Source: CAD feature listing. Evaluate the final solid. Frame: model axes, mm. Face numbers are marked on the shaded views. A direction names the side the tool comes from. Coordinates: 2 decimals unless noted, no trailing zeros. Order: outer loops, then holes, each group sorted by start corner. A loop starts at its lowest first (then second) coordinate and runs counter-clockwise, first axis right, second up.
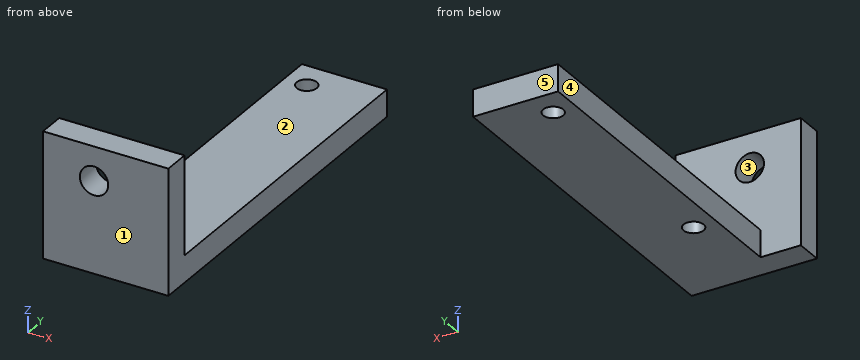
```python
from build123d import *

# Parameters (mm, degrees)
SKETCH1_W               = 10
SKETCH1_H               = 10
SKETCH1_H_2             = 65
SKETCH1_R               = 2.25
BOSS_EXTRUDE1_DEPTH     = 6
SKETCH2_W               = 28
SKETCH2_H               = 28
SKETCH2_R               = 3.175
BOSS_EXTRUDE2_DEPTH     = 6
SKETCH3_W               = 6
SKETCH3_H               = 75
BOSS_EXTRUDE3_DEPTH     = 9
SKETCH4_W               = 54.205081497
SKETCH4_H               = 103.631562047
CUT_EXTRUDE1_DEPTH      = 23
CUT_EXTRUDE1_DEPTH_BACK = 7


with BuildPart() as part:
    # Sketch1 → Boss-Extrude1 (new body)
    with BuildSketch(Plane.XY):
        with Locations((0, -37.5)):
            Rectangle(SKETCH1_W, SKETCH1_H)
        Rectangle(SKETCH1_W, SKETCH1_H_2)
        with Locations((0, 26)):
            Circle(SKETCH1_R, mode=Mode.SUBTRACT)
        with Locations((0, -26)):
            Circle(SKETCH1_R, mode=Mode.SUBTRACT)
    extrude(amount=BOSS_EXTRUDE1_DEPTH)



with BuildPart() as body_2:
    # Sketch2 → Boss-Extrude2 (new body)
    with BuildSketch(Plane.XZ.offset(42.5)):
        with Locations((0, 14)):
            Rectangle(SKETCH2_W, SKETCH2_H)
        with Locations((2.6, 20.429948245)):
            Circle(SKETCH2_R, mode=Mode.SUBTRACT)
    extrude(amount=BOSS_EXTRUDE2_DEPTH)


with BuildPart() as part_1:
    add(part.part)

    add(body_2.part)  # Boss-Extrude3 merges body 2
    # Sketch3 → Boss-Extrude3 (add)
    with BuildSketch(Plane.ZY.offset(5)):
        with Locations((3, -5)):
            Rectangle(SKETCH3_W, SKETCH3_H)
    extrude(amount=BOSS_EXTRUDE3_DEPTH)

    # Mirror1: part across plane


with BuildPart() as part_2:
    add(part_1.part)
    add(part_1.part.mirror(Plane(origin=(-14, -48.5, 0), x_dir=(0, 0, 1), z_dir=(-1, 0, 0))))

    # Sketch4 → Cut-Extrude1 (cut, two sides)
    with BuildSketch(Plane.XY.offset(6)) as cut_extrude1_sk:
        with Locations((13.102540749, -19.315781024)):
            Rectangle(SKETCH4_W, SKETCH4_H)
    extrude(amount=CUT_EXTRUDE1_DEPTH, mode=Mode.SUBTRACT)
    extrude(cut_extrude1_sk.sketch, amount=-CUT_EXTRUDE1_DEPTH_BACK, mode=Mode.SUBTRACT)


solid = part_2.part
```
1. Section query A-A, the plane y = -26. Output: boundary loops of the cut face in (x, z).
2. Contact query for flat-ended pins moving along their axis: P1, Ø2, axis at x = -17.5, y = 22.5, coming from the -Z side; P2, Ø9.5, axis at x = -23, y = -1, coming from the +Z side; P3, Ø12, axis at y = -31.5, z = 5.5, coming from the -X side. Output: stop coordinate, or through.
3. Section query B-B, the plane z = 22.25. Output: boundary loops of the cut face in (x, y).
4. Section query D-D, the plane x = -24.5. Output: boundary loops of the cut face in (y, z).
5. Draft query along X for the marked faces 3, 4 and 5. Return one class per face: +X half, -X half, draft (parallel to the pull), parting line (faces both ways), or undercut.
6. Section query C-C, the plane x = -28.5. Output: boundary loops of the cut face in (y, z).
7. Material intervals for line 1 along Y through (x, z) = (-28, 1.3); line 2 along Z through (x, y) = (-30.6, -46.6); line 3 along Y through (x, z) = (-26.25, 5.5), sorted ascending.
8. Access query for the marked faces 1 and 2. Directions: +Z, -Z, +X, -X, +Y, -Y. A direction counts if a zero-diameter tool reaches every point of the face in a straight line with its end or side. Return the directions, or none.
Answer key:
1. outline: (-33, 0) - (-30.25, 0) - (-30.25, 6) - (-33, 6) - close; (-25.75, 0) - (-14, 0) - (-14, 6) - (-25.75, 6) - close
2. P1: stops at z = 0
2. P2: stops at z = 6
2. P3: stops at x = -33
3. outline: (-42, -48.5) - (-33.2, -48.5) - (-33.2, -42.5) - (-42, -42.5) - close; (-28, -48.5) - (-14, -48.5) - (-14, -42.5) - (-28, -42.5) - close
4. outline: (-48.5, 0) - (32.5, 0) - (32.5, 6) - (-42.5, 6) - (-42.5, 28) - (-48.5, 28) - close
5. face 3: undercut
5. face 4: -X half
5. face 5: draft
6. outline: (-48.5, 0) - (-28.19, 0) - (-28.19, 6) - (-42.5, 6) - (-42.5, 18.05) - (-48.5, 18.05) - close; (-48.5, 22.81) - (-42.5, 22.81) - (-42.5, 28) - (-48.5, 28) - close; (-23.81, 0) - (23.81, 0) - (23.81, 6) - (-23.81, 6) - close; (28.19, 0) - (32.5, 0) - (32.5, 6) - (28.19, 6) - close
7. line 1: y = -48.5 to -28.25, -23.75 to 23.75, 28.25 to 32.5
7. line 2: z = 0 to 17.25, 23.6 to 28
7. line 3: y = -48.5 to -27.41, -24.59 to 24.59, 27.41 to 32.5
8. face 1: +Z, -Z, +X, -X, -Y
8. face 2: +Z, +X, -X, +Y
